```python
from build123d import *

# Parameters (mm, degrees)
BOSS_EXTRUDE1_DEPTH     = 35
CUT_EXTRUDE4_DEPTH      = 52.815716631
CUT_EXTRUDE4_DEPTH_BACK = 52.815716631
SKETCH6_R               = 1.4732
CUT_EXTRUDE5_DEPTH      = 53.815781867
CUT_EXTRUDE5_DEPTH_BACK = 53.815781867
SKETCH7_R               = 1.4732
CUT_EXTRUDE6_DEPTH      = 54.018864735
CUT_EXTRUDE7_DEPTH      = 42.163897972
CUT_EXTRUDE8_DEPTH      = 8.255
CUT_EXTRUDE9_DEPTH      = 0.254


with BuildPart() as part:
    # Sketch1 → Boss-Extrude1 (new body)
    with BuildSketch(Plane.XY):
        with BuildLine():
            Line((-35, 0), (-35, -19))
            ThreePointArc((-35, -19), (-17.5, -17.653892856), (0, -19))
            Line((0, -19), (0, 0))
            Line((0, 0), (-35, 0))
        make_face()
    extrude(amount=BOSS_EXTRUDE1_DEPTH)

    # Sketch6 → Cut-Extrude4 (cut, two sides: drawn at the far end of the back side and taken through both)
    with BuildSketch(Plane(origin=(-1.62776516, -18.605440918, 0), x_dir=(0.9961946980917455, -0.08715574274765824, 0), z_dir=(-0.08715574274765824, -0.9961946980917455, 0)).offset(-CUT_EXTRUDE4_DEPTH_BACK)):
        with Locations((-5.932999587, 29.70276)):
            Circle(SKETCH6_R)
    extrude(amount=CUT_EXTRUDE4_DEPTH + CUT_EXTRUDE4_DEPTH_BACK, mode=Mode.SUBTRACT)

    # Sketch7 → Cut-Extrude5 (cut, two sides: drawn at the far end of the back side and taken through both)
    with BuildSketch(Plane(origin=(1.361900838, -15.566597809, 0), x_dir=(0.9961946980917455, 0.08715574274765851, 0), z_dir=(0.08715574274765851, -0.9961946980917455, 0)).offset(-CUT_EXTRUDE5_DEPTH_BACK)):
        with Locations((-28.933814846, 29.70276)):
            Circle(SKETCH7_R)
    extrude(amount=CUT_EXTRUDE5_DEPTH + CUT_EXTRUDE5_DEPTH_BACK, mode=Mode.SUBTRACT)

    # Sketch8 → Cut-Extrude6 (cut, through all)
    with BuildSketch(Plane(origin=(0, 0, 0), x_dir=(-1, 0, 0), z_dir=(0, 0, -1))):
        with BuildLine():
            ThreePointArc((0, -7.571999996), (17.5, -6.224379342), (35, -7.571999996))
            Line((35, -7.571999996), (35, 0))
            Line((35, 0), (0, 0))
            Line((0, 0), (0, -7.571999996))
        make_face()
    extrude(amount=-CUT_EXTRUDE6_DEPTH, mode=Mode.SUBTRACT)

    # Sketch9 → Cut-Extrude7 (cut, through all)
    with BuildSketch(Plane(origin=(-17.5, -6.224379342, 0), x_dir=(-1, 0, 0), z_dir=(0, 1, 0))):
        with BuildLine():
            ThreePointArc((0, 15.85), (-3, 12.85), (0, 9.85))
            Line((0, 9.85), (0, 15.85))
        make_face()
        with BuildLine():
            Line((0, 15.85), (0, 9.85))
            ThreePointArc((0, 9.85), (2.121320344, 10.728679656), (3, 12.85))
            ThreePointArc((3, 12.85), (2.121320344, 14.971320344), (0, 15.85))
        make_face()
    extrude(amount=-CUT_EXTRUDE7_DEPTH, mode=Mode.SUBTRACT)

    # Sketch9_3 → Cut-Extrude8 (cut)
    with BuildSketch(Plane(origin=(-17.5, -6.224379342, 0), x_dir=(-1, 0, 0), z_dir=(0, 1, 0))):
        with BuildLine():
            ThreePointArc((0, 17.215625), (-4.365625, 12.85), (0, 8.484375))
            Line((0, 8.484375), (0, 9.85))
            ThreePointArc((0, 9.85), (-3, 12.85), (0, 15.85))
            Line((0, 15.85), (0, 17.215625))
        make_face()
        with BuildLine():
            Line((0, 9.85), (0, 8.484375))
            ThreePointArc((0, 8.484375), (3.086963042, 9.763036958), (4.365625, 12.85))
            ThreePointArc((4.365625, 12.85), (3.086963042, 15.936963042), (0, 17.215625))
            Line((0, 17.215625), (0, 15.85))
            ThreePointArc((0, 15.85), (2.121320344, 14.971320344), (3, 12.85))
            ThreePointArc((3, 12.85), (2.121320344, 10.728679656), (0, 9.85))
        make_face()
    extrude(amount=-CUT_EXTRUDE8_DEPTH, mode=Mode.SUBTRACT)

    # Sketch9_4 → Cut-Extrude9 (cut)
    with BuildSketch(Plane(origin=(-17.5, -6.224379342, 0), x_dir=(-1, 0, 0), z_dir=(0, 1, 0))):
        with BuildLine():
            ThreePointArc((0, 20.47), (-7.62, 12.85), (0, 5.23))
            Line((0, 5.23), (0, 8.484375))
            ThreePointArc((0, 8.484375), (-4.365625, 12.85), (0, 17.215625))
            Line((0, 17.215625), (0, 20.47))
        make_face()
        with BuildLine():
            Line((0, 8.484375), (0, 5.23))
            ThreePointArc((0, 5.23), (5.388153673, 7.461846327), (7.62, 12.85))
            ThreePointArc((7.62, 12.85), (5.388153673, 18.238153673), (0, 20.47))
            Line((0, 20.47), (0, 17.215625))
            ThreePointArc((0, 17.215625), (3.086963042, 15.936963042), (4.365625, 12.85))
            ThreePointArc((4.365625, 12.85), (3.086963042, 9.763036958), (0, 8.484375))
        make_face()
    extrude(amount=-CUT_EXTRUDE9_DEPTH, mode=Mode.SUBTRACT)


solid = part.part
```
Check sheet for the modelled part. Datum: model origin and axes. Units: mm. A direction names the side the tool comes from. Give positions to 0.01 mm unless a question says otherwise; leave off trailing zeros. Order: outer loops, then holes, each group sorted by start corner. A loop starts at its lowest first (then second) coordinate and runs counter-clockwise, first axis right, second up. Notation, with made-up numbers: M 48.25,-10 L 67.25,-10 A21 ccw 67.25,20 Z; hole C -35.75,-39 d2. An arc over 180 degrees is marked long. Answer in a Markdown table with one row per item. Add a question column.
Q1. Sectioned sample at D-D, the plane y = -8.75. Count the separate pieces of the cut face and the enclosed holes in it, and give its area (3 significant figures).
Q2. Thickness scan on L1, parallel to X at y = -14, z = 11; L2, parallel to X at y = -16.5, z = 28.5; L3, parallel to X at y = -13, z = 13. Record the ranges inside material, lowest first.
Q3. Sectioned sample at A-A, the plane x = -16.5. Record the boundary of the cut face in (y, z).
Q4. Access from +Z, -Z, +X, -X, +Y, -Y to the whole of each face (thin tool, end or side, straight path). Record for faces 4 (the cylindrical face through (-17.746, -17.654, 17.255)), 5 (the flat face through (-16, -14.479, 10)).
Q5. Sectioned sample at C-C, the plane z = 26. Record the boundary of the cut face in (x, y), and give its area (3 significant figures).
Q6. Release check for a two-part mould opening along Z. For faces 1 (the flat face through (-18, -13, 35)), 2 (the cylindrical face through (-29.43, -12.47, 29.77)), 3 (the flat face through (0, -13, 17)) record: released by +Z, released by -Z, zero draft, split by the parting line, or undercut.
Q7. Gauge pin test, flat ends, axial feed: pin 1 Ø6 at (x, z) = (-18.5, 16.5) entering from -Y; pin 2 Ø9.5 at (x, z) = (-15.5, 14) entering from +Y; pin 3 Ø4 at (x, z) = (-21, 9.5) entering from -Y. Record the tip position at first contact, or that the pin passes through.
Verdict:
| question | item | result |
|---|---|---|
| 1 | separate pieces | 1 |
| 1 | enclosed holes | 3 |
| 1 | area | 1,150 mm² |
| 2 | L1 | -35 to -21.45, -13.55 to 0 |
| 2 | L2 | -35 to -28.45, -26.75 to -8.25, -6.55 to 0 |
| 2 | L3 | -35 to -21.86, -13.14 to 0 |
| 3 | outline | M -17.66,0 L -6.23,0 L -6.23,5.3 L -6.48,5.3 L -6.48,8.6 L -14.48,8.6 L -14.48,10.02 L -17.66,10.02 Z; M -17.66,15.68 L -14.48,15.68 L -14.48,17.1 L -6.48,17.1 L -6.48,20.4 L -6.23,20.4 L -6.23,35 L -17.66,35 Z |
| 4 | face 4 | +Z, -Z, -Y |
| 4 | face 5 | +Y |
| 5 | outline | M -35,-19 A114.43 cw 0,-19 L 0,-7.57 A114.3 ccw -35,-7.57 Z |
| 5 | area | 400 mm² |
| 6 | face 1 | released by +Z |
| 6 | face 2 | undercut |
| 6 | face 3 | zero draft |
| 7 | pin 1 | y = -17.72 |
| 7 | pin 2 | y = -6.48 |
| 7 | pin 3 | y = -17.79 |
